Can you work these out from the model? Positions are in its coordinate system, mm. A direction names the side the tool comes from. Give positions to 0.01 mm unless a question says otherwise; leave off trailing zeros. Order: outer loops, then holes, each group sorted by start corner. A loop starts at its lowest first (then second) coordinate and runs counter-clockwise, first axis right, second up. Notation, with made-up numbers: (19, 7.5) - (77, 7.5) arc R12 cw to (77, 22.5) - close; hole circle Ø5 at (83, -3.5). An arc over 180 degrees is marked (long way). Answer as a JSON object with one key per item and string values.
```python
from build123d import *

# Parameters (mm, degrees)
F0_W     = 4.5
F0_H     = 25
F1_DEPTH = 1000
F2_R     = 7.5
F3_DEPTH = 125
F4_W     = 48
F4_H     = 39.5
F5_DEPTH = 10
F7_DEPTH = 50
F9_DEPTH = 34.501
F11_D    = 11


with BuildPart() as f1:
    # F0 (on Top) → F1 (new body)
    with BuildSketch(Plane.XY):
        Polygon((2.25, -2.25), (19, -2.25), (19, 2.25), (-19, 2.25), (-19, -2.25), (-2.25, -2.25), align=None)
        with Locations((0, -14.75)):
            Rectangle(F0_W, F0_H)
    extrude(amount=F1_DEPTH)

    # F2 (on Right) → F3 (join, symmetric)
    with BuildSketch(Plane.YZ):
        with Locations((-14.75, 850)):
            Circle(F2_R)
    extrude(amount=F3_DEPTH, both=True)

    # F4 (on face) → F5 (join)
    with BuildSketch(Plane.XY.offset(1000)):
        with Locations((0, -12.5)):
            Rectangle(F4_W, F4_H)
    extrude(amount=F5_DEPTH)

    # F6 (on Right) → F7 (cut, symmetric)
    with BuildSketch(Plane.YZ):
        Polygon((-27.25, 0), (2.25, 0), (-27.25, 51.0954988233), align=None)
    extrude(amount=F7_DEPTH, both=True, mode=Mode.SUBTRACT)

    # F8 (on face) → F9 (cut, through all)
    with BuildSketch(Plane(origin=(0, 2.25, 0), x_dir=(-1, 0, 0), z_dir=(0, 1, 0))):
        Polygon((-19, 0), (0, 0), (-19, 52.2020709696), align=None)
        Polygon((19, 52.2020709696), (0, 0), (19, 0), align=None)
    extrude(amount=-F9_DEPTH, mode=Mode.SUBTRACT)

    # F11 (through all)
    with Locations(Plane.YZ.offset(2.25)):
        with Locations((-14.75, 925)):
            Hole(F11_D / 2)


solid = f1.part
```
Q1. If we section it at B-B, the plane x = -107: Please give me the cut outline in (y, z).
Recorded:
{"outline": "circle Ø15 at (-14.75, 850)"}
Q2. I need wall thicknesses on L1, parallel to Y at x = 0, z = 925; L2, parallel to Y at x = 17.5, z = 768. Which ranges of each line are inside material? Lowest first, please.
Recorded:
{"L1": "y = -27.25 to -20.25, -9.25 to 2.25", "L2": "y = -2.25 to 2.25"}
Q3. We'd pull the mould along Z, two halves only. Please class faces 1 (the face through (0, -12, 1010)), 2 (the face through (11, -2.25, 497)), 3 (the face through (5, -12, 1000)): released by +Z, released by -Z, zero draft, split by the parting line, or undercut.
Recorded:
{"face 1": "released by +Z", "face 2": "zero draft", "face 3": "undercut"}
Q4. I'm going to push flat-ended pins straight in: pin 1 Ø9 at (y, z) = (-14.75, 925) entering from -X; pin 2 Ø19 at (x, z) = (-9.5, 315.5) entering from +Y; pin 3 Ø11 at (y, z) = (-4, 1003) entering from +X; pin 4 Ø5 at (y, z) = (1, 470.5) entering from +X. Where does each tip first touch, or does it pass through?
Recorded:
{"pin 1": "passes through", "pin 2": "stops at y = 2.25", "pin 3": "stops at x = 24", "pin 4": "stops at x = 19"}
Q5. Which directions (+Z, -Z, +X, -X, +Y, -Y) give clear straight access to the entire face, cutting with the end or side of a thin tool? Please do faces 4 (the face through (0, 2.25, 493)), 5 (the face through (0, -12.3, 25.2)).
Recorded:
{"face 4": "-Z, +X, -X, +Y", "face 5": "-Z, +X, -X, -Y"}
Q6. If we section it at A-A, the plane z = 188: Please give me the cut outline in (x, y).
Recorded:
{"outline": "(-19, -2.25) - (-2.25, -2.25) - (-2.25, -27.25) - (2.25, -27.25) - (2.25, -2.25) - (19, -2.25) - (19, 2.25) - (-19, 2.25) - close"}
